Answer from the drawing. Dimensions are ordinates in mm from the lowest x, y and z of the part. A direction names the side the tool comes from. Round coordinates to 2 decimals unless told otherwise and drop trailing zeros. Write each loop counter-clockwise with the first axis right and the second up, starting at its lowest first coordinate (ties: lowest second). Pieces come first, ordered by that corner, then holes. Notation, with made-up numbers: M -31,64 L 26,64 A24 cw 26,78 Z; hole C 22.5,-13 d1. An arc over 180 degrees is marked long. Answer as CSV lines item,"result". Start each with the question number.
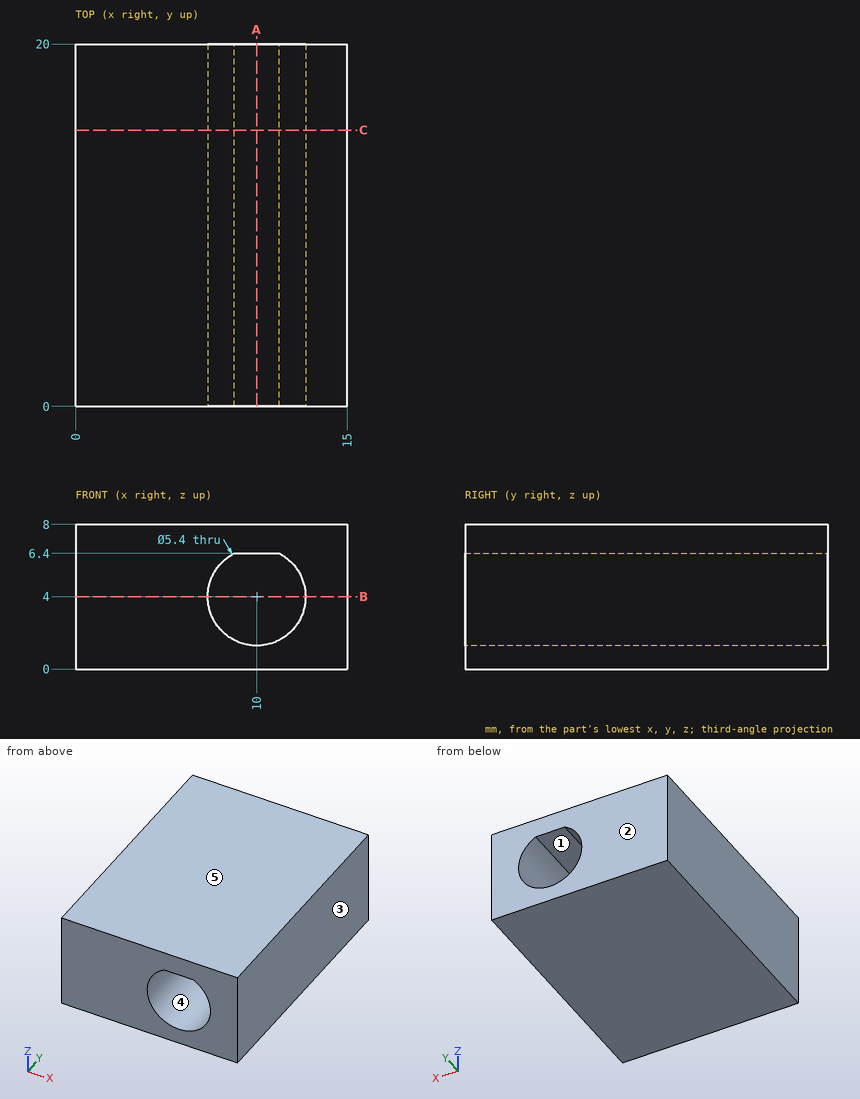
Q1. Find section B-B (z = 4). Determine the outline of the cut face in (x, y), plus the area to 3 significant figures.
Q2. Find section C-C (y = 15.25). Determine the outline of the cut face in (x, z).
Q3. This flat-tipped pin is pushed along its axis until it touches: P1, Ø3, axis at x = 8, z = 6.5, coming from the -Y side. Where does it stop, or does it pass through?
Q4. The mould has two halves that part along X. Classify the marked faces 3, 4 and 5: +X half, -X half, draft (parallel to the pull), parting line (faces both ways), or undercut.
Q5. Find section A-A (x = 10). Determine the outline of the cut face in (y, z), plus the area to 3 significant figures.
Q6. For the marked faces 1 and 2, determine the directions among +Z, -Z, +X, -X, +Y, -Y from which every point of the face is accessible in a straight line to the end or side of a thin tool.
Q7. Straight lines are drawn through the part: L1, parallel to Z at x = 10, y = 6.5; L2, parallel to X at y = 13.5, z = 4; L3, parallel to Z at x = 12, y = 10. For each, find the intervals that lie inside material, in ascending order.
Reported:
1,outline,"M 0,0 L 7.3,0 L 7.3,20 L 0,20 Z; M 12.7,0 L 15,0 L 15,20 L 12.7,20 Z"
1,area,"192 mm2"
2,outline,"M 0,0 L 15,0 L 15,8 L 0,8 Z; hole M 8.76,6.4 A2.7 ccw long 11.24,6.4 Z"
3,P1,"stops at y = 0"
4,face 3,"+X half"
4,face 4,"undercut"
4,face 5,"draft"
5,outline,"M 0,0 L 20,0 L 20,1.3 L 0,1.3 Z; M 0,6.4 L 20,6.4 L 20,8 L 0,8 Z"
5,area,"58.0 mm2"
6,face 1,"+Y, -Y"
6,face 2,"+Z, -Z, +X, -X, +Y"
7,L1,"z = 0 to 1.3, 6.4 to 8"
7,L2,"x = 0 to 7.3, 12.7 to 15"
7,L3,"z = 0 to 2.19, 5.81 to 8"
